Answer from the drawing. Dimensions are ordinates in mm from the lowest x, y and z of the part. Coordinates: 2 decimals unless noted, no trailing zeros. Loops run counter-clockwise (first coordinate to the right, second up) from the corner with the lowest first, then second, coordinate; pieces in that order, holes last. Notation, with made-up numbers: (14, 81) - (25, 81) arc R6 ccw to (25, 91) - close; hole circle Ø10 at (48.5, 6). An arc over 180 degrees is marked (long way). Write each question's results on one line, items separated by ' | '. Start each with the question number.
1. Find the intervals of material crossed by line 1 along Z through (x, y) = (12.35, 6.25) (3 decimals); line 2 along X through (y, z) = (9, 14), in increasing order. Write a range as [from, to].
2. A cutting plane is placed at A-A on z = 14. Determine the outline of the cut face in (x, y).
3. A cutting plane is placed at B-B on y = 15. Determine the outline of the cut face in (x, z) (3 decimals), then the cut area to 3 significant figures.
4. A cutting plane is placed at C-C on x = 12.35. Determine the outline of the cut face in (y, z) (3 decimals).
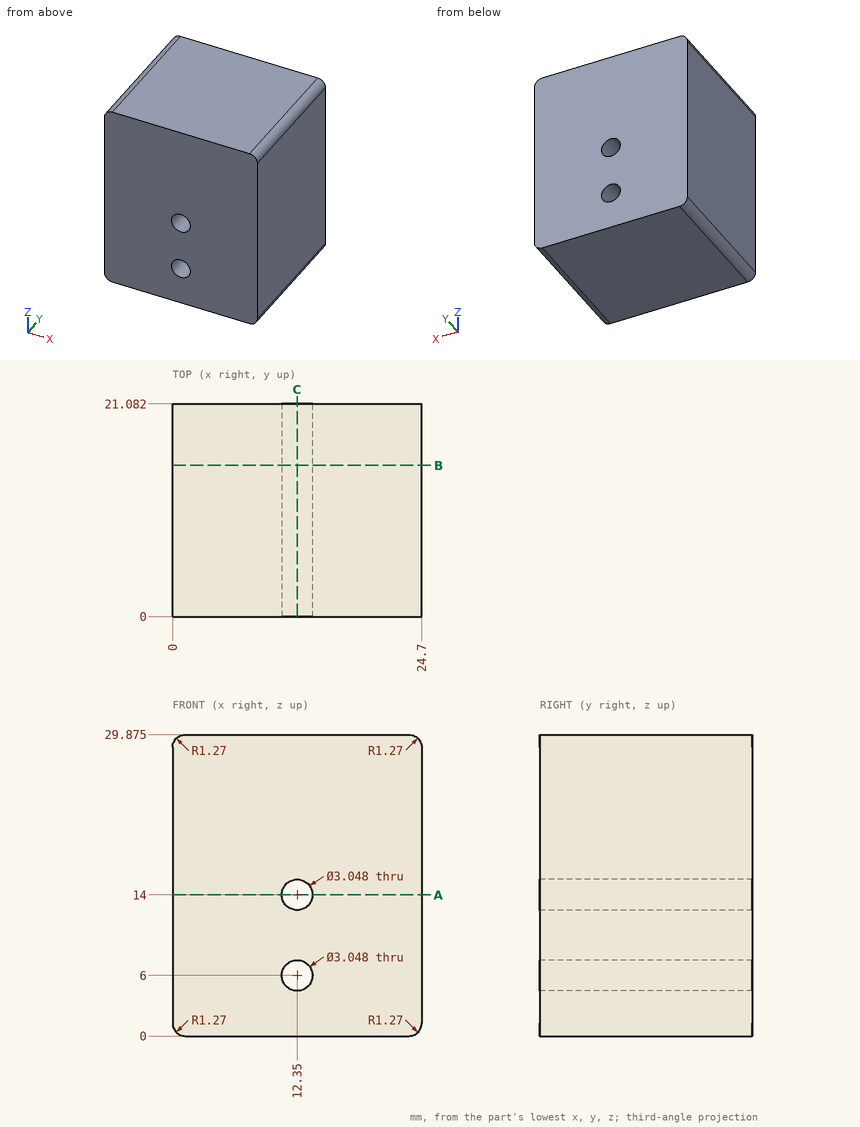
Values:
1) line 1: [0, 4.476], [7.524, 12.476], [15.524, 29.875] | line 2: [0, 10.83], [13.87, 24.7]
2) outline: (0, 0) - (10.83, 0) - (10.83, 21.08) - (0, 21.08) - close; (13.87, 0) - (24.7, 0) - (24.7, 21.08) - (13.87, 21.08) - close
3) outline: (0, 1.27) arc R1.27 ccw to (1.27, 0) - (23.43, 0) arc R1.27 ccw to (24.7, 1.27) - (24.7, 28.605) arc R1.27 ccw to (23.43, 29.875) - (1.27, 29.875) arc R1.27 ccw to (0, 28.605) - close; hole circle Ø3.048 at (12.35, 6); hole circle Ø3.048 at (12.35, 14) | area: 722 mm^2
4) outline: (0, 0) - (21.082, 0) - (21.082, 4.476) - (0, 4.476) - close; (0, 7.524) - (21.082, 7.524) - (21.082, 12.476) - (0, 12.476) - close; (0, 15.524) - (21.082, 15.524) - (21.082, 29.875) - (0, 29.875) - close
